Work out the finished part from the listing and answer in its coordinate system (mm). Face numbers are marked on the shaded views. Coordinates: 2 decimals unless noted, no trailing zeros. Write each loop counter-clockwise with the first axis right and the second up, starting at its lowest first coordinate (ties: lowest second). Pieces come first, ordered by that corner, then holes. Notation, with made-up numbers: (-33, -1) -> (4, -1) arc R8 cw to (4, 9) -> close; hole circle Ø4 at (78.25, -28.75). An arc over 180 degrees is marked (long way). Write each question's results on one line, items separated by ' | '. Start each with the question number.
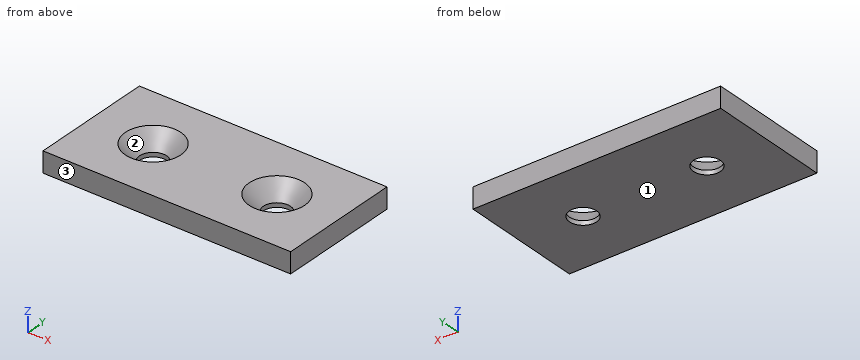
from build123d import *

# Parameters (mm, degrees)
SKETCH1_W                    = 76.2
SKETCH1_H                    = 38.1
SKETCH1_R                    = 4.1656
BOSS_EXTRUDE1_DEPTH          = 3.175
CUT_EXTRUDE1_START           = -5.0292
SKETCH2_R                    = 4.1656
CUT_EXTRUDE1_DEPTH           = 91.459712699
CUT_EXTRUDE1_DRAFT           = -41
CUT_EXTRUDE1_PROFILE_2_DEPTH = 91.459712699
CUT_EXTRUDE1_PROFILE_2_DRAFT = -41


with BuildPart() as part:
    # Sketch1 → Boss-Extrude1 (new, symmetric)
    with BuildSketch(Plane.XY):
        with Locations((38.1, 19.05)):
            Rectangle(SKETCH1_W, SKETCH1_H)
        with Locations((19.05, 19.05)):
            Circle(SKETCH1_R, mode=Mode.SUBTRACT)
        with Locations((57.15, 19.05)):
            Circle(SKETCH1_R, mode=Mode.SUBTRACT)
    extrude(amount=BOSS_EXTRUDE1_DEPTH, both=True)


with BuildPart() as cut_extrude1_tool:
    # Sketch2 → Cut-Extrude1 (with draft: the straight prism first)
    with BuildSketch(Plane.XY.offset(3.175).offset(CUT_EXTRUDE1_START)):
        with Locations((19.05, 19.05)):
            Circle(SKETCH2_R)
    extrude(amount=CUT_EXTRUDE1_DEPTH)
    # Cut-Extrude1: the draft: its side faces are tilted about the plane it starts from
    cut_extrude1_sides = [cut_extrude1_tool.faces().sort_by_distance(p)[0] for p in [
        (14.8844, 19.05, 43.875656349),
    ]]
    draft(cut_extrude1_sides, Plane.XY.offset(3.175).offset(CUT_EXTRUDE1_START), CUT_EXTRUDE1_DRAFT)


with BuildPart() as part_1:
    add(part.part)

    # Cut-Extrude1: cut by cut_extrude1_tool
    add(cut_extrude1_tool.part, mode=Mode.SUBTRACT)


with BuildPart() as cut_extrude1_profile_2_tool:
    # Sketch2 → Cut-Extrude1 profile 2 (with draft: the straight prism first)
    with BuildSketch(Plane.XY.offset(3.175).offset(CUT_EXTRUDE1_START)):
        with Locations((57.15, 19.05)):
            Circle(SKETCH2_R)
    extrude(amount=CUT_EXTRUDE1_PROFILE_2_DEPTH)
    # Cut-Extrude1 profile 2: the draft: its side faces are tilted about the plane it starts from
    cut_extrude1_profile_2_sides = [cut_extrude1_profile_2_tool.faces().sort_by_distance(p)[0] for p in [
        (52.9844, 19.05, 43.875656349),
    ]]
    draft(cut_extrude1_profile_2_sides, Plane.XY.offset(3.175).offset(CUT_EXTRUDE1_START), CUT_EXTRUDE1_PROFILE_2_DRAFT)


with BuildPart() as part_2:
    add(part_1.part)

    # Cut-Extrude1 profile 2: cut by cut_extrude1_profile_2_tool
    add(cut_extrude1_profile_2_tool.part, mode=Mode.SUBTRACT)


solid = part_2.part
1. Find the intervals of material crossed by L1, parallel to Y at x = 57.15, z = -2.8; L2, parallel to X at y = 20, z = 0.75; L3, parallel to X at y = 13, z = 1, in increasing order.
2. Find section C-C on z = 0. Give the vertices of the cut face in (x, y), and give its area (3 significant figures).
3. Given pin 1 Ø7.5 at (x, y) = (19.05, 19.05) entering from -Z; pin 2 Ø13.5 at (x, y) = (57.15, 19.05) entering from +Z, each flat-ended and moving along its own axis, determine where each tip first touches the part or whether it passes through.
4. Find section A-A on x = 57.15. Give the vertices of the cut face in (y, z) (3 decimals), and give its area (3 significant figures).
5. Determine the mould class of the marked faces 1, 2 and 3 for opening direction Y: pulls with the +Y half, pulls with the -Y half, needs draft (parallel to the pull), parting line crosses it, or undercut.
6. Find section B-B on y = 19.05. Give the vertices of the cut face in (x, z) (3 decimals).
Ans:
1) L1: y = 0 to 14.88, 23.22 to 38.1 | L2: x = 0 to 12.69, 25.41 to 50.79, 63.51 to 76.2 | L3: x = 0 to 16.3, 21.8 to 54.4, 59.9 to 76.2
2) outline: (0, 0) -> (76.2, 0) -> (76.2, 38.1) -> (0, 38.1) -> close; hole circle Ø11.55 at (19.05, 19.05); hole circle Ø11.55 at (57.15, 19.05) | area: 2,690 mm²
3) pin 1: passes through | pin 2: stops at z = 1.12
4) outline: (0, -3.175) -> (14.884, -3.175) -> (14.884, -1.854) -> (10.513, 3.175) -> (0, 3.175) -> close; (23.216, -3.175) -> (38.1, -3.175) -> (38.1, 3.175) -> (27.587, 3.175) -> (23.216, -1.854) -> close | area: 167 mm²
5) face 1: needs draft | face 2: undercut | face 3: pulls with the -Y half
6) outline: (0, -3.175) -> (14.884, -3.175) -> (14.884, -1.854) -> (10.513, 3.175) -> (0, 3.175) -> close; (23.216, -3.175) -> (52.984, -3.175) -> (52.984, -1.854) -> (48.613, 3.175) -> (27.587, 3.175) -> (23.216, -1.854) -> close; (61.316, -3.175) -> (76.2, -3.175) -> (76.2, 3.175) -> (65.687, 3.175) -> (61.316, -1.854) -> close
